Input: dimensioned drawing with shaded views. Units: mm. Origin: part minimum x, y, z. Coordinates: 2 decimals unless noted, no trailing zeros. Order: outer loops, then holes, each group sorted by start corner. A loop starts at its lowest first (then second) coordinate and runs counter-clockwise, first axis right, second up. Notation, with made-up numbers: (19, 48.25) -> (54, 48.25) arc R32 cw to (54, 77.25) -> close; hole circle Ø3 at (58.5, 65.25). An arc over 180 degrees is marked (long way). Put each result on its own line as item: value.
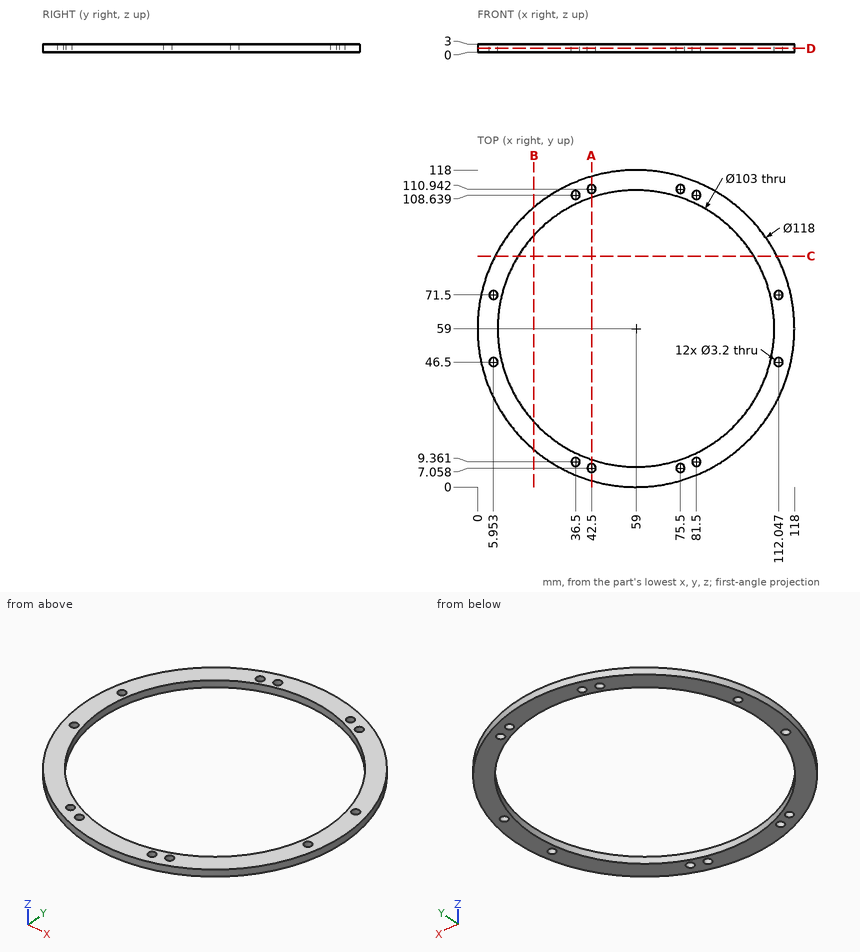
1. Ray query, line 1 along X through (y, z) = (6, 2.75) (1 decimal); line 2 along X through (y, z) = (71.5, 2.2); line 3 along X through (y, z) = (72.5, 0.65) (1 decimal). Return the intervals inside material, ascending.
Numbers:
line 1: x = 33.1 to 41.3, 43.7 to 74.3, 76.7 to 84.9
line 2: x = 1.34 to 4.35, 7.55 to 9.04, 108.96 to 110.45, 113.65 to 116.66
line 3: x = 1.6 to 4.7, 7.2 to 9.3, 108.7 to 110.8, 113.3 to 116.4
2. First-contact query: pin 1 (3 mm diameter, centred on x = 75.5, y = 110.94, fed in from -Z); pin 2 (1.5 mm diameter, centred on x = 12.5, z = 2, fed in from +Y) (1 decimal). Flat tips, straight axial feed; report the tip coordinate or a pass-through.
Numbers:
pin 1: passes through
pin 2: stops at y = 96.3
3. Cut plane C-C on y = 86. Output: boundary loops of the cut face in (x, z) (1 decimal).
Numbers:
outline: (6.5, 0) -> (15.1, 0) -> (15.1, 3) -> (6.5, 3) -> close; (102.9, 0) -> (111.5, 0) -> (111.5, 3) -> (102.9, 3) -> close
4. Cut plane D-D on z = 1.4. Count the separate pieces of the cut face and the enclosed holes in it, plus the area to 3 significant figures.
Numbers:
separate pieces: 1
enclosed holes: 13
area: 2,510 mm2
5. Cut plane B-B on x = 21. Output: boundary loops of the cut face in (y, z).
Numbers:
outline: (13.87, 0) -> (24.24, 0) -> (24.24, 3) -> (13.87, 3) -> close; (93.76, 0) -> (104.13, 0) -> (104.13, 3) -> (93.76, 3) -> close
6. Cut plane A-A on x = 42.5. Output: boundary loops of the cut face in (y, z) (1 decimal).
Numbers:
outline: (2.4, 0) -> (5.5, 0) -> (5.5, 3) -> (2.4, 3) -> close; (8.7, 0) -> (10.2, 0) -> (10.2, 3) -> (8.7, 3) -> close; (107.8, 0) -> (109.3, 0) -> (109.3, 3) -> (107.8, 3) -> close; (112.5, 0) -> (115.6, 0) -> (115.6, 3) -> (112.5, 3) -> close
